```python
from build123d import *

# Parameters (mm, degrees)
SKETCH1_R           = 6.35
SKETCH1_R_2         = 6.321908291
BOSS_EXTRUDE1_DEPTH = 38.1


with BuildPart() as part:
    # Sketch1 → Boss-Extrude1 (new body)
    with BuildSketch(Plane.XY):
        with BuildLine():
            Line((25.4632885, -63.5), (152.4, -63.5))
            ThreePointArc((152.4, -63.5), (161.380256121, -59.780256121), (165.1, -50.8))
            Line((165.1, -50.8), (165.1, -25.442050481))
            ThreePointArc((165.1, -25.442050481), (168.819743879, -16.46179436), (177.8, -12.742050481))
            ThreePointArc((177.8, -12.742050481), (190.5, -0.042050481), (177.8, 12.657949519))
            ThreePointArc((177.8, 12.657949519), (168.735231625, 16.383513436), (164.910134501, 25.406732606))
            Line((164.910134501, 25.406732606), (164.910134501, 50.8632885))
            ThreePointArc((164.910134501, 50.8632885), (161.208927395, 59.798792893), (152.273423001, 63.5))
            Line((152.273423001, 63.5), (25.3367115, 63.5))
            ThreePointArc((25.3367115, 63.5), (16.356455379, 59.780256121), (12.6367115, 50.8))
            Line((12.6367115, 50.8), (12.6367115, 25.406732606))
            ThreePointArc((12.6367115, 25.406732606), (9.016254993, 16.402760527), (0.0632885, 12.657949519))
            ThreePointArc((0.0632885, 12.657949519), (-12.6367115, -0.042050481), (0.0632885, -12.742050481))
            ThreePointArc((0.0632885, -12.742050481), (9.043544621, -16.46179436), (12.7632885, -25.442050481))
            Line((12.7632885, -25.442050481), (12.7632885, -50.8))
            ThreePointArc((12.7632885, -50.8), (16.483032379, -59.780256121), (25.4632885, -63.5))
        make_face()
        with Locations(Location((0, 0, 0), (0, 0, 180))):
            Circle(SKETCH1_R, mode=Mode.SUBTRACT)
        with Locations(Location((177.8, 0, 0), (0, 0, 180))):
            Circle(SKETCH1_R, mode=Mode.SUBTRACT)
        with Locations(Location((88.9, 50.8, 0), (0, 0, 180))):
            Circle(SKETCH1_R, mode=Mode.SUBTRACT)
        with Locations(Location((88.9, -50.8, 0), (0, 0, 180))):
            Circle(SKETCH1_R, mode=Mode.SUBTRACT)
        with Locations(Location((152.3367115, 50.8, 0), (0, 0, 180))):
            Circle(SKETCH1_R_2, mode=Mode.SUBTRACT)
        with Locations(Location((25.4, 50.8, 0), (0, 0, 180))):
            Circle(SKETCH1_R, mode=Mode.SUBTRACT)
        with Locations(Location((25.4, -50.8, 0), (0, 0, 180))):
            Circle(SKETCH1_R, mode=Mode.SUBTRACT)
        with Locations(Location((152.3367115, -50.8, 0), (0, 0, 180))):
            Circle(SKETCH1_R, mode=Mode.SUBTRACT)
        with BuildLine():
            Line((34.925, 30.1625), (34.925, -30.1625))
            ThreePointArc((34.925, -30.1625), (36.784871939, -34.652628061), (41.275, -36.5125))
            Line((41.275, -36.5125), (136.525, -36.5125))
            ThreePointArc((136.525, -36.5125), (141.015128061, -34.652628061), (142.875, -30.1625))
            Line((142.875, -30.1625), (142.875, 30.1625))
            ThreePointArc((142.875, 30.1625), (141.015128061, 34.652628061), (136.525, 36.5125))
            Line((136.525, 36.5125), (41.275, 36.5125))
            ThreePointArc((41.275, 36.5125), (36.784871939, 34.652628061), (34.925, 30.1625))
        make_face(mode=Mode.SUBTRACT)
    extrude(amount=BOSS_EXTRUDE1_DEPTH)


solid = part.part
```
For this review, take the finished solid that the model builds, in its own axes (mm). A direction names the side the tool comes from. Give positions to 0.01 mm unless a question says otherwise; leave off trailing zeros. Loops run counter-clockwise (first coordinate to the right, second up) from the corner with the lowest first, then second, coordinate; pieces in that order, holes last. Notation, with made-up numbers: M 18.5,28.5 L 39.5,28.5 A9 cw 39.5,43.5 Z; hole C 1,12 d2. An arc over 180 degrees is marked long. One line per item, written item: value. Start each with the question number.
Q1. For L1, parallel to X at y = 50.8, z = 14; L2, parallel to X at y = -50.8, z = 9.5; L3, parallel to Y at x = 120, z = 10, list the stretches that pass through material, from the lowest coordinate up.
Q2. Add section D-D (x = 112). Give the boundary of the cut face in (y, z), and give its area (3 significant figures).
Q3. Add section B-B (x = 88.9). Give the boundary of the cut face in (y, z), and give its area (3 significant figures).
Q4. Add section A-A (y = -28). Give the boundary of the cut face in (x, z) (3 decimals).
Q5. Draft analysis for pull direction X (two halves, no side actions). For faces 4 (the face through (90, 63.5, 19)), 5 (the face through (146.28, -52.71, 18.78)), 6 (the face through (26.2, -57.1, 18.8)), 7 (the face through (164.91, 38, 19)), state which applies: released by +X, released by -X, zero draft, split by the parting line, or undercut.
Q6. Machinability: for faces 1 (the face through (12.763, -38, 19)), 2 (the face through (88, -63.5, 19)), 3 (the face through (141.064, 34.603, 18.783)), which of the approach directions +Z, -Z, +X, -X, +Y, -Y give a long, thin tool a straight path to every point of the face, cutting with its end or side? Answer none if there is none.
Q7. Add section C-C (z = 10). Count the separate pieces of the cut face and the enclosed holes in it, and give its area (3 significant figures).
Q8. Clearance check with flat-ended pins moving along their axes: pin 1 Ø12.5 at (y, z) = (-34, 18.5) entering from +X; pin 2 Ø11.5 at (y, z) = (-8.5, 10) entering from -X; pin 3 Ø7.5 at (y, z) = (-32.5, 11.5) entering from -X. State where each tip first meets the part, or that it passes through.
Reply:
1. L1: 12.64 to 19.05, 31.75 to 82.55, 95.25 to 146.01, 158.66 to 164.91
1. L2: 12.76 to 19.05, 31.75 to 82.55, 95.25 to 145.99, 158.69 to 165.1
1. L3: -63.5 to -36.51, 36.51 to 63.5
2. outline: M -63.5,0 L -36.51,0 L -36.51,38.1 L -63.5,38.1 Z; M 36.51,0 L 63.5,0 L 63.5,38.1 L 36.51,38.1 Z
2. area: 2,060 mm²
3. outline: M -63.5,0 L -57.15,0 L -57.15,38.1 L -63.5,38.1 Z; M -44.45,0 L -36.51,0 L -36.51,38.1 L -44.45,38.1 Z; M 36.51,0 L 44.45,0 L 44.45,38.1 L 36.51,38.1 Z; M 57.15,0 L 63.5,0 L 63.5,38.1 L 57.15,38.1 Z
3. area: 1,090 mm²
4. outline: M 12.763,0 L 34.925,0 L 34.925,38.1 L 12.763,38.1 Z; M 142.875,0 L 165.1,0 L 165.1,38.1 L 142.875,38.1 Z
5. face 4: zero draft
5. face 5: undercut
5. face 6: undercut
5. face 7: released by +X
6. face 1: +Z, -Z, -X, -Y
6. face 2: +Z, -Z, +X, -X, -Y
6. face 3: +Z, -Z
7. separate pieces: 1
7. enclosed holes: 9
7. area: 11,600 mm²
8. pin 1: x = 165.1
8. pin 2: x = -12.34
8. pin 3: x = 12.76
